from build123d import *

# Parameters (mm, degrees)
SKETCH2_W            = 15.8
SKETCH2_H            = 15.8
BOSS_EXTRUDE2_DEPTH  = 4.2
SKETCH4_W            = 13.4
SKETCH4_H            = 13.4
CUT_EXTRUDE1_DEPTH   = 3
SKETCH6_R            = 2.41
BOSS_EXTRUDE4_DEPTH  = 1.8
LPATTERN1_COUNT      = 2
LPATTERN1_PITCH      = 8
LPATTERN1_COUNT_DIR2 = 2
LPATTERN1_PITCH_DIR2 = 8
SKETCH8_R            = 5.25
CUT_EXTRUDE2_DEPTH   = 0.1
BOSS_EXTRUDE9_DEPTH  = 3
CUT_EXTRUDE3_DEPTH   = 3
CIRPATTERN3_COUNT    = 4


with BuildPart() as part:
    # Sketch2 → Boss-Extrude2 (new body)
    with BuildSketch(Plane(origin=(0, 0, 0), x_dir=(1, 0, 0), z_dir=(0, 1, 0))):
        with Locations((7.9, 7.9)):
            Rectangle(SKETCH2_W, SKETCH2_H)
    extrude(amount=-BOSS_EXTRUDE2_DEPTH)

    # Sketch4 → Cut-Extrude1 (cut)
    with BuildSketch(Plane(origin=(0, 0, 0), x_dir=(1, 0, 0), z_dir=(0, 1, 0))):
        with Locations((7.9, 7.9)):
            Rectangle(SKETCH4_W, SKETCH4_H)
    extrude(amount=-CUT_EXTRUDE1_DEPTH, mode=Mode.SUBTRACT)

    # Sketch6 → Boss-Extrude4 (add)
    with BuildSketch(Plane(origin=(0, -4.2, 0), x_dir=(-1, 0, 0), z_dir=(0, -1, 0))):
        with Locations((-11.9, 11.9)):
            Circle(SKETCH6_R)
    boss_extrude4 = extrude(amount=BOSS_EXTRUDE4_DEPTH)

    # LPattern1: Boss-Extrude4 2 × 2
    with Locations(*[(-j * LPATTERN1_PITCH_DIR2, 0, i * LPATTERN1_PITCH) for i in range(LPATTERN1_COUNT) for j in range(LPATTERN1_COUNT_DIR2) if (i, j) != (0, 0)]):
        add(boss_extrude4)

    # Sketch8 → Cut-Extrude2 (cut)
    with BuildSketch(Plane(origin=(0, -3, 0), x_dir=(1, 0, 0), z_dir=(0, 1, 0))):
        with Locations((7.9, 7.9)):
            Circle(SKETCH8_R)
    extrude(amount=-CUT_EXTRUDE2_DEPTH, mode=Mode.SUBTRACT)

    # Sketch11 → Boss-Extrude9 (add)
    with BuildSketch(Plane(origin=(0, -3, 0), x_dir=(1, 0, 0), z_dir=(0, 1, 0))):
        with BuildLine():
            Line((7.899999971, 14.6), (1.2, 14.6))
            Line((1.2, 14.6), (1.2, 7.9))
            ThreePointArc((1.2, 7.9), (3.162384556, 12.637615424), (7.899999971, 14.6))
        make_face()
        with BuildLine():
            Line((14.6, 14.6), (7.899999971, 14.6))
            ThreePointArc((7.899999971, 14.6), (12.637615424, 12.637615444), (14.6, 7.9))
            Line((14.6, 7.9), (14.6, 14.6))
        make_face()
        with BuildLine():
            ThreePointArc((7.900000011, 1.2), (3.16238457, 3.162384562), (1.2, 7.9))
            Line((1.2, 7.9), (1.2, 1.2))
            Line((1.2, 1.2), (7.900000011, 1.2))
        make_face()
        with BuildLine():
            Line((14.6, 1.2), (14.6, 7.9))
            ThreePointArc((14.6, 7.9), (12.637615438, 3.16238457), (7.900000011, 1.2))
            Line((7.900000011, 1.2), (14.6, 1.2))
        make_face()
    extrude(amount=BOSS_EXTRUDE9_DEPTH)

    # Sketch12 → Cut-Extrude3 (cut)
    with BuildSketch(Plane(origin=(0, 0, 0), x_dir=(1, 0, 0), z_dir=(0, 1, 0))):
        Polygon((3.162384566, 12.637615434), (2.031013716, 13.768986284), (0.970353544, 12.708326112), (2.101724394, 11.576955262), align=None)
        with BuildLine():
            ThreePointArc((2.221981276, 11.45669838), (2.658816927, 12.073727351), (3.162384566, 12.637615434))
            Line((3.162384566, 12.637615434), (2.101724394, 11.576955262))
            Line((2.101724394, 11.576955262), (2.221981276, 11.45669838))
        make_face()
        with BuildLine():
            Line((4.223044738, 13.698275606), (3.162384566, 12.637615434))
            ThreePointArc((3.162384566, 12.637615434), (3.726272649, 13.141183073), (4.34330162, 13.578018724))
            Line((4.34330162, 13.578018724), (4.223044738, 13.698275606))
        make_face()
        Polygon((3.091673888, 14.829646456), (2.031013716, 13.768986284), (3.162384566, 12.637615434), (4.223044738, 13.698275606), align=None)
        with BuildLine():
            ThreePointArc((4.34330162, 13.578018724), (3.726272649, 13.141183073), (3.162384566, 12.637615434))
            ThreePointArc((3.162384566, 12.637615434), (2.658816927, 12.073727351), (2.221981276, 11.45669838))
            Line((2.221981276, 11.45669838), (2.423581348, 11.255098309))
            Line((2.423581348, 11.255098309), (4.544901691, 13.376418652))
            Line((4.544901691, 13.376418652), (4.34330162, 13.578018724))
        make_face()
        with BuildLine():
            ThreePointArc((14.6, 7.9), (11.145005458, 13.761735202), (4.34330162, 13.578018724))
            Line((4.34330162, 13.578018724), (4.544901691, 13.376418652))
            Line((4.544901691, 13.376418652), (2.423581348, 11.255098309))
            Line((2.423581348, 11.255098309), (2.221981276, 11.45669838))
            ThreePointArc((2.221981276, 11.45669838), (6.049692654, 1.460561925), (14.6, 7.9))
        make_face()
    cut_extrude3 = extrude(amount=-CUT_EXTRUDE3_DEPTH, mode=Mode.SUBTRACT)

    # CirPattern3: Cut-Extrude3 ×4 about axis
    cirpattern3_axis = Axis((7.9, 0, -7.9), (0, 1, 0))
    for i in range(1, CIRPATTERN3_COUNT):
        add(cut_extrude3.rotate(cirpattern3_axis, i * 360 / CIRPATTERN3_COUNT), mode=Mode.SUBTRACT)


solid = part.part
Work out the finished part from the listing and answer in its coordinate system (mm). A direction names the side the tool comes from. Give positions to 0.01 mm unless a question says otherwise; leave off trailing zeros. Loops run counter-clockwise (first coordinate to the right, second up) from the corner with the lowest first, then second, coordinate; pieces in that order, holes last. Notation, with made-up numbers: (-36.75, 49.5) -> (8.25, 49.5) arc R24 cw to (8.25, 88.5) -> close; hole circle Ø7 at (8.25, -24.75). An arc over 180 degrees is marked (long way). Use a Markdown table: item, result. Add a question column.
1) The part is cut by section C-C, the plane x = 12.5. Determine the outline of the cut face in (y, z).
2) The part is cut by section A-A, the plane y = -1.85. Determine the outline of the cut face in (x, z).
3) Consider line 1 along Z through (x, y) = (11.75, -5.15); line 2 along Y through (x, z) = (10, -9.75); line 3 along Y through (x, z) = (12.75, -13.25). Determine where each line is inside the solid, lowest interval first.
4) The part is cut by section B-B, the plane z = -2. Determine the outline of the cut face in (x, y), plus the area to 3 significant figures.
5) Which of the six approach directions +Z, -Z, +X, -X, +Y, -Y give full straight-line access (tool end or side, diameter ignored) to faces 1 (the cylindrical face through (2.79, -5.09, -9.76)), 2 (the flat face through (15.8, -2, -8)), 3 (the flat face through (13.784, -1.479, -13.754))?
6) Each of these flat-tipped pins is pushed along its axis until it touches: P1, Ø3, axis at x = 10, z = -6.5, coming from the +Y side; P2, Ø4, axis at x = 6, z = -11, coming from the +Y side. Where does it stop, or does it pass through?
7) The part is cut by section D-D, the plane y = -5.15. Determine the outline of the cut face in (x, z), plus the area to 3 significant figures.
8) For a pull along Z with two mould halves and no side action, classify faces 4 (the cylindrical face through (12.422, -5.087, -9.547)), 5 (the flat face through (12, -6, -4)), 6 (the flat face through (8, -2, 0)) as +Z half, -Z half, draft (parallel to the pull), parting line (faces both ways), or undercut.
Reported:
| question | item | result |
|---|---|---|
| 1 | outline | (-6, -14.23) -> (-4.2, -14.23) -> (-4.2, -15.8) -> (0, -15.8) -> (0, -14.62) -> (-3, -14.62) -> (-3, -10.43) -> (-3.1, -10.43) -> (-3.1, -5.37) -> (-3, -5.37) -> (-3, -1.18) -> (0, -1.18) -> (0, 0) -> (-4.2, 0) -> (-4.2, -1.57) -> (-6, -1.57) -> (-6, -6.23) -> (-4.2, -6.23) -> (-4.2, -9.57) -> (-6, -9.57) -> close |
| 2 | outline | (0, -15.8) -> (15.8, -15.8) -> (15.8, 0) -> (0, 0) -> close; hole (0.97, -12.71) -> (3.09, -14.83) -> (4.34, -13.58) arc R6.7 ccw to (11.46, -13.58) -> (12.71, -14.83) -> (14.83, -12.71) -> (13.58, -11.46) arc R6.7 ccw to (13.58, -4.34) -> (14.83, -3.09) -> (12.71, -0.97) -> (11.46, -2.22) arc R6.7 ccw to (4.34, -2.22) -> (3.09, -0.97) -> (0.97, -3.09) -> (2.22, -4.34) arc R6.7 ccw to (2.22, -11.46) -> close |
| 3 | line 1 | z = -14.31 to -9.49, -6.31 to -1.49 |
| 3 | line 2 | y = -4.2 to -3.1 |
| 3 | line 3 | y = -6 to -3 |
| 4 | outline | (0, -4.2) -> (2.42, -4.2) -> (2.42, -6) -> (5.38, -6) -> (5.38, -4.2) -> (10.42, -4.2) -> (10.42, -6) -> (13.38, -6) -> (13.38, -4.2) -> (15.8, -4.2) -> (15.8, 0) -> (13.74, 0) -> (13.74, -3) -> (11.68, -3) -> (11.68, 0) -> (11.07, 0) -> (11.07, -3) -> (4.73, -3) -> (4.73, 0) -> (4.12, 0) -> (4.12, -3) -> (2.06, -3) -> (2.06, 0) -> (0, 0) -> close |
| 4 | area | 45.6 mm^2 |
| 5 | face 1 | -Y |
| 5 | face 2 | +Z, -Z, +X, +Y, -Y |
| 5 | face 3 | +Y |
| 6 | P1 | stops at y = -3.1 |
| 6 | P2 | stops at y = -3 |
| 7 | outline | circle Ø4.82 at (3.9, -11.9); circle Ø4.82 at (3.9, -3.9); circle Ø4.82 at (11.9, -11.9); circle Ø4.82 at (11.9, -3.9) |
| 7 | area | 73.0 mm^2 |
| 8 | face 4 | undercut |
| 8 | face 5 | draft |
| 8 | face 6 | +Z half |
